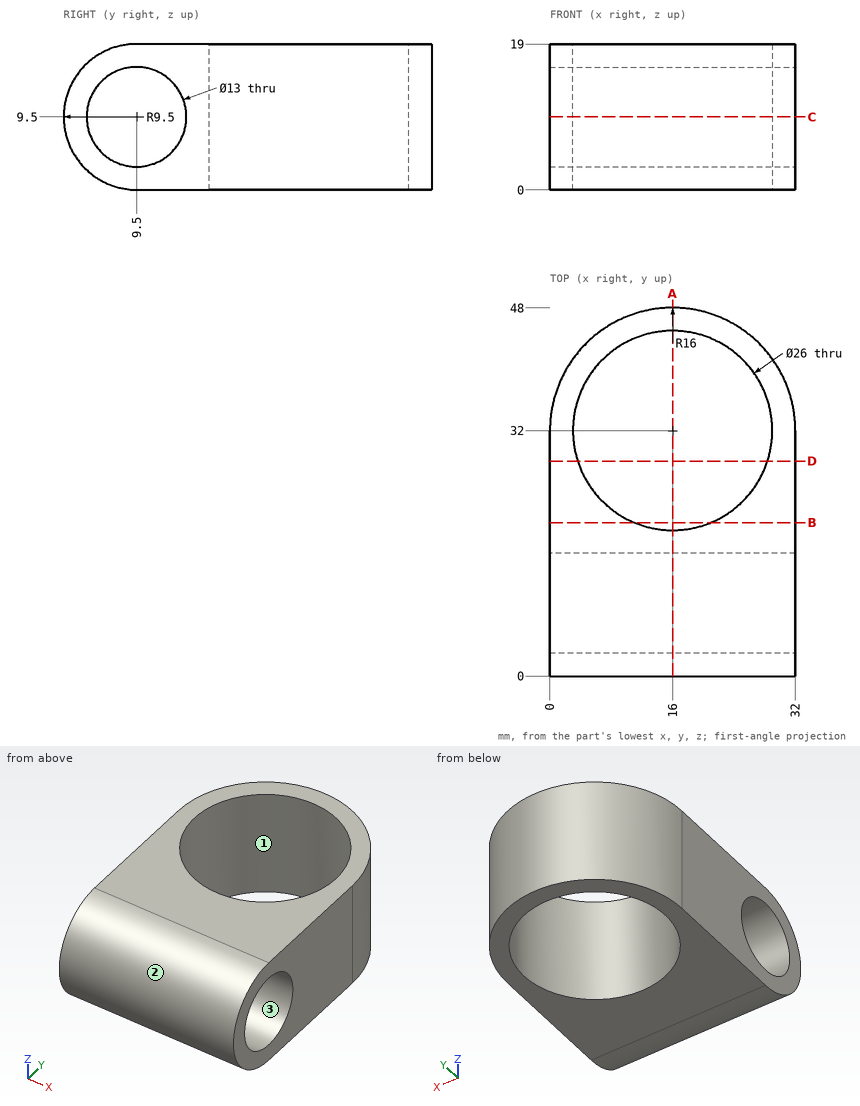
Print and shaded views of the part. All mm, measured from the part's lowest x, y and z. Coordinates: 2 decimals unless noted, no trailing zeros. Order: outer loops, then holes, each group sorted by start corner. A loop starts at its lowest first (then second) coordinate and runs counter-clockwise, first axis right, second up. Notation, with made-up numbers: (54.25, -19) -> (85.25, -19) arc R14 ccw to (85.25, -8) -> close; hole circle Ø1 at (-28.75, -33). An arc over 180 degrees is marked (long way). Use one line per item in the form item = value. Start each with the question number.
1) Band-saw the part on B-B on y = 20. Give the cut face in (x, z).
2) Band-saw the part on D-D on y = 28. Give the cut face in (x, z), then the cut area to 3 significant figures.
3) Band-saw the part on C-C on z = 9.5. Give the cut face in (x, y), then the cut area to 3 significant figures.
4) Pull direction Z, two halves, no side cores. Call the marked faces 1, 2 and 3: +Z half, -Z half, draft (parallel to the pull), parting line (faces both ways), or undercut.
5) Band-saw the part on A-A on x = 16. Give the cut face in (y, z).
6) Drill centre lines: L1, parallel to Y at x = 15, z = 9.75; L2, parallel to Y at x = 16, z = 5.5; L3, parallel to Z at x = 22.5, y = 9.5. Where is each one in solid material? Low to high. Write a range as [from, to].
7) Drop flat-ended pins along their axis: pin 1 (8 mm diameter, centred on y = 42, z = 15, fed in from -X); pin 2 (5 mm diameter, centred on x = 19.5, z = 5, fed in from +Y); pin 3 (1 mm diameter, centred on x = 12, z = 13.5, fed in from -Y); pin 4 (10.5 mm diameter, centred on y = 9.5, z = 9.5, fed in from -X). Give the stop position or say it passes through.
Entries:
q1.outline = (0, 0) -> (11, 0) -> (11, 19) -> (0, 19) -> close; (21, 0) -> (32, 0) -> (32, 19) -> (21, 19) -> close
q2.outline = (0, 0) -> (3.63, 0) -> (3.63, 19) -> (0, 19) -> close; (28.37, 0) -> (32, 0) -> (32, 19) -> (28.37, 19) -> close
q2.area = 138 mm2
q3.outline = (0, 0) -> (32, 0) -> (32, 3) -> (0, 3) -> close; (0, 16) -> (32, 16) -> (32, 32) arc R16 ccw to (0, 32) -> close; hole circle Ø26 at (16, 32)
q3.area = 479 mm2
q4.face_1 = draft
q4.face_2 = parting line
q4.face_3 = undercut
q5.outline = (9.5, 0) -> (19, 0) -> (19, 19) -> (9.5, 19) arc R9.5 ccw to start; (45, 0) -> (48, 0) -> (48, 19) -> (45, 19) -> close; hole circle Ø13 at (9.5, 9.5)
q6.L1 = [0, 3], [16, 19.04], [44.96, 47.97]
q6.L2 = [0.88, 4.38], [14.62, 19], [45, 48]
q6.L3 = [0, 3], [16, 19]
q7.pin_1 = 1.17
q7.pin_2 = 47.97
q7.pin_3 = 0.67
q7.pin_4 = through
